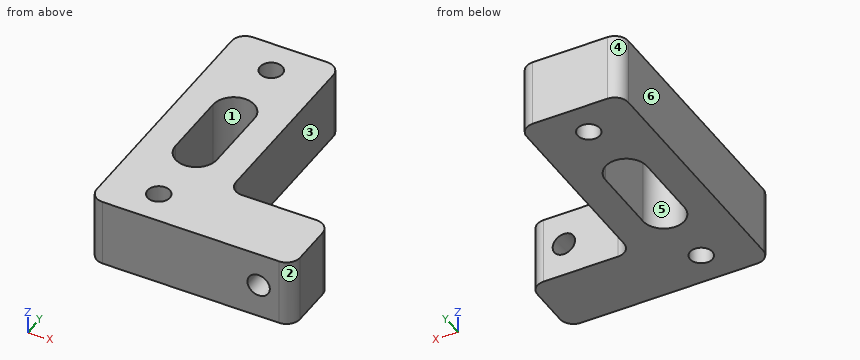
from build123d import *

# Parameters (mm, degrees)
SKETCH_1_R          = 1.65
EXTRUDE_1_DEPTH     = 10
SKETCH_5_R          = 1.65
CUT_EXTRUDE_2_DEPTH = 10
BODY_CUT_DEPTH      = 10
FILLET_1_R          = 2
FILLET_2_R          = 2


with BuildPart() as part:
    # ｽｹｯﾁ1 → ﾎﾞｽ - 押し出し1 (new body)
    with BuildSketch(Plane.XY):
        Polygon((0, 0), (0, -40), (30, -40), (30, -30), (15, -30), (15, 0), align=None)
        with Locations((7.5, -5)):
            Circle(SKETCH_1_R, mode=Mode.SUBTRACT)
        with Locations((7.5, -35)):
            Circle(SKETCH_1_R, mode=Mode.SUBTRACT)
    extrude(amount=EXTRUDE_1_DEPTH)

    # ｽｹｯﾁ5 → ｶｯﾄ - 押し出し2 (cut)
    with BuildSketch(Plane.XZ.offset(40)):
        with Locations(Location((25, 5, 0), (0, 0, 270))):
            Circle(SKETCH_5_R)
    extrude(amount=-CUT_EXTRUDE_2_DEPTH, mode=Mode.SUBTRACT)

    # ｽｹｯﾁ7 → body cut (cut)
    with BuildSketch(Plane.XY.offset(10)):
        with BuildLine():
            Line((10.55, -15), (10.55, -25))
            ThreePointArc((10.55, -25), (7.5, -28.05), (4.45, -25))
            Line((4.45, -25), (4.45, -15))
            ThreePointArc((4.45, -15), (7.5, -11.95), (10.55, -15))
        make_face()
    extrude(amount=-BODY_CUT_DEPTH, mode=Mode.SUBTRACT)

    # ﾌｨﾚｯﾄ1
    fillet_1_edges = [part.edges().sort_by_distance(p)[0] for p in [
        (15, -30, 5),
    ]]
    fillet(fillet_1_edges, radius=FILLET_1_R)

    # ﾌｨﾚｯﾄ2
    fillet_2_edges = [part.edges().sort_by_distance(p)[0] for p in [
        (15, 0, 5),
        (30, -30, 5),
        (30, -40, 5),
        (0, -40, 5),
        (0, 0, 5),
    ]]
    fillet(fillet_2_edges, radius=FILLET_2_R)


solid = part.part
Geometry: final body of the model. Coordinates: model frame, mm. Face numbers are marked on the shaded views. A direction names the side the tool comes from. Coordinates: 2 decimals unless noted, no trailing zeros. Order: outer loops, then holes, each group sorted by start corner. A loop starts at its lowest first (then second) coordinate and runs counter-clockwise, first axis right, second up.
1) First-contact query: P1, Ø4, axis at x = 7.5, y = -35, coming from the -Z side; P2, Ø5, axis at x = 22.5, z = 4, coming from the +Y side; P3, Ø5, axis at y = -28.5, z = 8.5, coming from the +X side; P4, Ø5, axis at y = -4.5, z = 2, coming from the +X side. Flat tips, straight axial feed; report the tip coordinate or a pass-through.
Result sheet:
P1: stops at z = 0
P2: stops at y = -30
P3: stops at x = 29.73
P4: stops at x = 15
2) Section B-B (x = 7.5). Return loops of the section in (y, z).
Result sheet:
outline: (-40, 0) - (-36.65, 0) - (-36.65, 10) - (-40, 10) - close; (-33.35, 0) - (-28.05, 0) - (-28.05, 10) - (-33.35, 10) - close; (-11.95, 0) - (-6.65, 0) - (-6.65, 10) - (-11.95, 10) - close; (-3.35, 0) - (0, 0) - (0, 10) - (-3.35, 10) - close
3) Section C-C (y = -5). Return loops of the section in (x, z).
Result sheet:
outline: (0, 0) - (5.85, 0) - (5.85, 10) - (0, 10) - close; (9.15, 0) - (15, 0) - (15, 10) - (9.15, 10) - close
4) Draft query along Y for the marked faces 4, 5 and 6. Return one class per face: released by +Y, released by -Y, zero draft, split by the parting line, or undercut.
Result sheet:
face 4: released by +Y
face 5: undercut
face 6: zero draft
5) Set-up query: the marked faces 1, 2 and 3. Return all of +Z, -Z, +X, -X, +Y, -Y with unobstructed straight access to the full face (end or side cutting, diameter ignored); none if empty.
Result sheet:
face 1: +Z, -Z
face 2: +Z, -Z, +X, -Y
face 3: +Z, -Z, +X, +Y
6) Section A-A (x = 25). Return loops of the section in (y, z).
Result sheet:
outline: (-40, 0) - (-30, 0) - (-30, 3.35) - (-40, 3.35) - close; (-40, 6.65) - (-30, 6.65) - (-30, 10) - (-40, 10) - close
7) Ray query, probe 1 along Y at (x, z) = (7.5, 3); probe 2 along Y at (x, z) = (9.75, 4); probe 3 along Y at (x, z) = (24.75, 2.75). Return the intervals inside material, ascending.
Result sheet:
probe 1: y = -40 to -36.65, -33.35 to -28.05, -11.95 to -6.65, -3.35 to 0
probe 2: y = -40 to -27.06, -12.94 to 0
probe 3: y = -40 to -30
8) Section D-D (z = 4). Return loops of the section in (x, y), then the cut area to 3 significant figures.
Result sheet:
outline: (0, -38) arc R2 ccw to (2, -40) - (23.69, -40) - (23.69, -30) - (17, -30) arc R2 cw to (15, -28) - (15, -2) arc R2 ccw to (13, 0) - (2, 0) arc R2 ccw to (0, -2) - close; (26.31, -40) - (28, -40) arc R2 ccw to (30, -38) - (30, -32) arc R2 ccw to (28, -30) - (26.31, -30) - close; hole (4.45, -25) arc R3.05 ccw to (10.55, -25) - (10.55, -15) arc R3.05 ccw to (4.45, -15) - close; hole circle Ø3.3 at (7.5, -35); hole circle Ø3.3 at (7.5, -5)
area: 613 mm2
